```python
from build123d import *

# Parameters (mm, degrees)
F0_R     = 3.175
F1_DEPTH = 9.525
F3_DEPTH = 127


with BuildPart() as f1:
    # F0 (on Front) → F1 (new body)
    with BuildSketch(Plane.XZ):
        with BuildLine():
            Line((-5.09987, 11.63105), (-3.99275, 12.056034))
            ThreePointArc((-3.99275, 12.056034), (-4.551273, 11.856471), (-5.09987, 11.63105))
        make_face()
        with BuildLine():
            Line((51.069545, 33.192469), (-3.99275, 12.056034))
            Line((-3.99275, 12.056034), (-5.09987, 11.63105))
            ThreePointArc((-5.09987, 11.63105), (-12.42989, -2.605347), (0, -12.7))
            Line((0, -12.7), (91.059, -12.7))
            ThreePointArc((91.059, -12.7), (98.425, -5.334), (91.059, 2.032))
            Line((91.059, 2.032), (71.374, 2.032))
            ThreePointArc((71.374, 2.032), (66.165451, 4.189451), (64.008, 9.398))
            Line((64.008, 9.398), (64.008, 24.300115))
            ThreePointArc((64.008, 24.300115), (59.878019, 32.149917), (51.069545, 33.192469))
        make_face()
        with BuildLine():
            ThreePointArc((5.715483, 4.505655), (9.555328, 8.254879), (13.335, 4.445))
            Line((13.335, 4.445), (13.335, -3.81))
            ThreePointArc((13.335, -3.81), (9.524889, -7.62), (5.715, -3.809779))
            Line((5.715, -3.809779), (5.715476, 4.384788))
            ThreePointArc((5.715476, 4.384788), (5.715, 4.445221), (5.715483, 4.505655))
        make_face(mode=Mode.SUBTRACT)
        with Locations((91.186, -5.334)):
            Circle(F0_R, mode=Mode.SUBTRACT)
        with BuildLine():
            ThreePointArc((40.64, 4.445), (44.45, 8.255), (48.26, 4.445))
            Line((48.26, 4.445), (48.26, -3.81))
            ThreePointArc((48.26, -3.81), (44.45, -7.62), (40.64, -3.81))
            Line((40.64, -3.81), (40.64, 4.445))
        make_face(mode=Mode.SUBTRACT)
        with Locations((53.975, 20.955)):
            Circle(F0_R, mode=Mode.SUBTRACT)
    extrude(amount=F1_DEPTH)

    # F2 (on face) → F3 (cut)
    with BuildSketch(Plane.XZ.offset(9.525)):
        with BuildLine():
            ThreePointArc((98.3742, -6.1976), (98.412289, -5.766546), (98.425, -5.334))
            Line((98.425, -5.334), (98.3742, -5.334))
            Line((98.3742, -5.334), (98.3742, -6.1976))
        make_face()
        with BuildLine():
            Line((98.3742, -5.334), (98.425, -5.334))
            ThreePointArc((98.425, -5.334), (98.412289, -4.901454), (98.3742, -4.4704))
            Line((98.3742, -4.4704), (98.3742, -5.334))
        make_face()
    extrude(amount=-F3_DEPTH, mode=Mode.SUBTRACT)


solid = f1.part
```
Can you work these out from the model? Positions are in its coordinate system, mm. A direction names the side the tool comes from. Coordinates: 2 decimals unless noted, no trailing zeros. Write each loop counter-clockwise with the first axis right and the second up, starting at its lowest first coordinate (ties: lowest second). Pieces come first, ordered by that corner, then holes. Notation, with made-up numbers: (-21.5, -4) - (-2.5, -4) arc R34 ccw to (-2.5, 29) - close; hole circle Ø2 at (31, 67). An arc over 180 degrees is marked (long way). Return JSON: item names as keys, results as strings.
Q1. On a 3-axis mill with a long thin cutter (end or side, diameter ignored), from which of +Z, -Z, +X, -X, +Y, -Y can I reach the whole of each face in a straight line? I mean faces 1 (the cylindrical face through (9.61, -4.7, -7.62)), 2 (the flat face through (81, -5, 2.032)), 3 (the cylindrical face through (59.98, -4.7, 32.08)). Say none if no direction works.
Computed values:
{"face 1": "+Y, -Y", "face 2": "+Z, +X, +Y, -Y", "face 3": "+Z, +Y, -Y"}
Q2. Thinking about a two-plate mould opening in X: for faces 4 (the cylindrical face through (-12.477, -4.696, -2.367)), 5 (the flat face through (45, -5, -12.7)), 6 (the cylindrical face through (50.803, -4.696, 21.095)), 7 (the cylindrical face through (66.223, -4.696, 4.132)), which applies, +X half, -X half, draft (parallel to the pull), parting line (faces both ways), or undercut?
Computed values:
{"face 4": "-X half", "face 5": "draft", "face 6": "undercut", "face 7": "+X half"}
Q3. If we section it at A-A (z = 23): Please give me the cut outline in (x, y) (3 decimals), then the cut area to 3 significant figures.
Computed values:
{"outline": "(24.517, -9.525) - (51.546, -9.525) - (51.546, 0) - (24.517, 0) - close; (56.404, -9.525) - (64.008, -9.525) - (64.008, 0) - (56.404, 0) - close", "area": "330 mm2"}
Q4. I'm going to push flat-ended pins straight in: pin 1 Ø4 at (y, z) = (-6.5, -7) entering from -X; pin 2 Ø1 at (y, z) = (-2.5, 26) entering from +X; pin 3 Ø3 at (y, z) = (-4.5, 18) entering from +X. Where does each tip first touch, or does it pass through?
Computed values:
{"pin 1": "stops at x = -11.67", "pin 2": "stops at x = 63.93", "pin 3": "stops at x = 64.01"}
Q5. If we section it at D-D (x = 83.5): Please give me the cut outline in (y, z) (3 decimals), then the cut area to 3 significant figures.
Computed values:
{"outline": "(-9.525, -12.7) - (0, -12.7) - (0, 2.032) - (-9.525, 2.032) - close", "area": "140 mm2"}
Q6. If we section it at B-B (x = 44.45): Please give me the cut outline in (y, z) (3 decimals).
Computed values:
{"outline": "(-9.525, -12.7) - (0, -12.7) - (0, -7.62) - (-9.525, -7.62) - close; (-9.525, 8.255) - (0, 8.255) - (0, 30.651) - (-9.525, 30.651) - close"}
Q7. Please list where these lines run through material, in increasing order: L1, parallel to X at y = -9, z = 4 (3 decimals); L2, parallel to X at y = -4.75, z = -1.5 (3 decimals); L3, parallel to Z at x = 56, y = -4.5. Write a range as from..to.
Computed values:
{"L1": "x = -12.054..5.715, 13.335..40.64, 48.26..66.362", "L2": "x = -12.611..5.715, 13.335..40.64, 48.26..97.349", "L3": "z = -12.7..18.51, 23.4..33.7"}
Q8. If we section it at C-C (y = -7): Please give me the cut outline in (x, z) (3 decimals).
Computed values:
{"outline": "(-5.1, 11.631) arc R12.7 ccw to (0, -12.7) - (91.059, -12.7) arc R7.366 ccw to (98.374, -6.198) - (98.374, -4.47) arc R7.366 ccw to (91.059, 2.032) - (71.374, 2.032) arc R7.366 cw to (64.008, 9.398) - (64.008, 24.3) arc R9.525 ccw to (51.07, 33.192) - (-3.993, 12.056) arc R12.7 ccw to start; hole (5.715, -3.81) arc R3.81 ccw to (13.335, -3.81) - (13.335, 4.445) arc R3.81 ccw to (5.715, 4.506) arc R3.809 ccw to (5.715, 4.385) - close; hole (40.64, -3.81) arc R3.81 ccw to (48.26, -3.81) - (48.26, 4.445) arc R3.81 ccw to (40.64, 4.445) - close; hole circle Ø6.35 at (53.975, 20.955); hole circle Ø6.35 at (91.186, -5.334)"}
